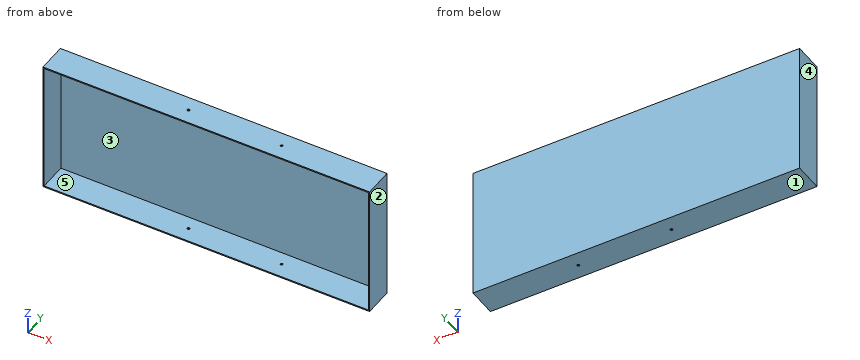
from build123d import *

# Parameters (mm, degrees)
F0_W     = 428.752
F0_H     = 175
F1_DEPTH = 38.1
F2_T     = -1.5875
F4_D     = 3.3


with BuildPart() as f1:
    # F0 (on Front) → F1 (new body)
    with BuildSketch(Plane.XZ):
        Rectangle(F0_W, F0_H)
    extrude(amount=F1_DEPTH)

    # F2
    f2_openings = [f1.faces().sort_by_distance(p)[0] for p in [
        (0, -38.1, 0),
    ]]
    offset(amount=F2_T, openings=f2_openings)

    # F4 (through all)
    with Locations(Plane(origin=(0, 0, -87.5), x_dir=(1, 0, 0), z_dir=(0, 0, -1))):
        with Locations((-34.8615, 19.05), (87.376, 19.05)):
            Hole(F4_D / 2)


solid = f1.part
Read the model definition and answer for the solid it produces. Units are mm, in the model's axes. Face numbers are marked on the shaded views. A direction names the side the tool comes from. Round coordinates to 2 decimals unless told otherwise and drop trailing zeros. Order: outer loops, then holes, each group sorted by start corner. A loop starts at its lowest first (then second) coordinate and runs counter-clockwise, first axis right, second up.
1) The part is cut by section C-C on z = -20. Write down the section's boundary in (x, y), plus the area to 3 significant figures.
2) The part is cut by section B-B on x = -129. Write down the section's boundary in (y, z), plus the area to 3 significant figures.
3) The part is cut by section A-A on y = -8.5. Write down the section's boundary in (x, z).
4) The mould has two halves that part along X. Classify the marked faces 1, 2 and 3: released by +X, released by -X, zero draft, split by the parting line, or undercut.
5) A flat-ended cylindrical pin translates along its axis: pin 1 (2 mm diameter, centred on x = 54, z = 41, fed in from -Y). Find the tip coordinate at first contact, or state that the pin passes through.
6) Straight lines are drawn through the part: L1, parallel to X at y = -19.05, z = 86.45; L2, parallel to X at y = -6.5, z = 13; L3, parallel to Z at x = 5, y = -22.5. For each, find the intervals that lie inside material, in ascending order.
7) For the marked faces 4 and 5, determine the directions among +Z, -Z, +X, -X, +Y, -Y from which every point of the face is accessible in a straight line to the end or side of a thin tool.
Resolved:
1. outline: (-214.38, -38.1) - (-212.79, -38.1) - (-212.79, -1.59) - (212.79, -1.59) - (212.79, -38.1) - (214.38, -38.1) - (214.38, 0) - (-214.38, 0) - close
1. area: 797 mm2
2. outline: (-38.1, -87.5) - (0, -87.5) - (0, 87.5) - (-38.1, 87.5) - (-38.1, 85.91) - (-1.59, 85.91) - (-1.59, -85.91) - (-38.1, -85.91) - close
2. area: 394 mm2
3. outline: (-214.38, -87.5) - (214.38, -87.5) - (214.38, 87.5) - (-214.38, 87.5) - close; hole (-212.79, -85.91) - (212.79, -85.91) - (212.79, 85.91) - (-212.79, 85.91) - close
4. face 1: zero draft
4. face 2: released by +X
4. face 3: undercut
5. pin 1: stops at y = -1.59
6. L1: x = -214.38 to -36.51, -33.21 to 85.73, 89.03 to 214.38
6. L2: x = -214.38 to -212.79, 212.79 to 214.38
6. L3: z = -87.5 to -85.91, 85.91 to 87.5
7. face 4: +Z, -Z, -X, +Y, -Y
7. face 5: -Y
